Design review of the part built by this model. Coordinates are the model's own, in mm. A direction names the side the tool comes from. Coordinates: 2 decimals unless noted, no trailing zeros. Loops run counter-clockwise (first coordinate to the right, second up) from the corner with the lowest first, then second, coordinate; pieces in that order, holes last. Notation, with made-up numbers: (-36.75, 22) - (-4.75, 22) arc R18 ccw to (-4.75, 47) - close; hole circle Ø4 at (-36, 56.5). An arc over 180 degrees is marked (long way). Return JSON: item names as keys, results as strings. Group by question number.
from build123d import *

# Parameters (mm, degrees)
F0_R      = 2.4509487717
F1_DEPTH  = 4.7244
F2_R      = 19.05
F3_DEPTH  = 1.524
F5_DEPTH  = 2.54
F7_DEPTH  = 5.842
F8_DEPTH  = 52.9844
F9_DEPTH  = 10.795
F10_R     = 2.032
F12_R     = 3.81
F13_DEPTH = 75.8698
F16_R     = 3.81
F17_DEPTH = 63.5
F18_R     = 3.175
F19_DEPTH = 25.4
F21_DEPTH = 11.5824


with BuildPart() as f1:
    # F0 (on Top) → F1 (new body)
    with BuildSketch(Plane.XY):
        with BuildLine():
            Line((25.273, 28.575), (-25.273, 28.575))
            ThreePointArc((-25.273, 28.575), (-27.6078665915, 27.6078665915), (-28.575, 25.273))
            Line((-28.575, 25.273), (-28.575, -25.273))
            ThreePointArc((-28.575, -25.273), (-27.6078665915, -27.6078665915), (-25.273, -28.575))
            Line((-25.273, -28.575), (25.273, -28.575))
            ThreePointArc((25.273, -28.575), (27.6078665915, -27.6078665915), (28.575, -25.273))
            Line((28.575, -25.273), (28.575, 25.273))
            ThreePointArc((28.575, 25.273), (27.6078665915, 27.6078665915), (25.273, 28.575))
        make_face()
        with Locations((-23.495, -23.495)):
            Circle(F0_R, mode=Mode.SUBTRACT)
        with Locations((23.495, -23.495)):
            Circle(F0_R, mode=Mode.SUBTRACT)
        with Locations((-23.495, 23.495)):
            Circle(F0_R, mode=Mode.SUBTRACT)
        with Locations((23.495, 23.495)):
            Circle(F0_R, mode=Mode.SUBTRACT)
    extrude(amount=-F1_DEPTH)

    # F2 (on face) → F3 (join)
    with BuildSketch(Plane(origin=(0, 0, -4.7244), x_dir=(1, 0, 0), z_dir=(0, 0, -1))):
        Circle(F2_R)
    extrude(amount=F3_DEPTH)

    # F4 (on face) → F5 (cut)
    with BuildSketch(Plane(origin=(0, 0, -4.7244), x_dir=(1, 0, 0), z_dir=(0, 0, -1))):
        with BuildLine():
            Line((-28.575, 12.7), (-25.019, 12.7))
            ThreePointArc((-25.019, 12.7), (-22.098, 15.621), (-25.019, 18.542))
            Line((-25.019, 18.542), (-28.575, 18.542))
            Line((-28.575, 18.542), (-28.575, 12.7))
        make_face()
        with BuildLine():
            Line((28.575, -12.7), (25.019, -12.7))
            ThreePointArc((25.019, -12.7), (22.098, -15.621), (25.019, -18.542))
            Line((25.019, -18.542), (28.575, -18.542))
            Line((28.575, -18.542), (28.575, -12.7))
        make_face()
        with BuildLine():
            Line((12.7, 28.575), (12.7, 25.019))
            ThreePointArc((12.7, 25.019), (15.621, 22.098), (18.542, 25.019))
            Line((18.542, 25.019), (18.542, 28.575))
            Line((18.542, 28.575), (12.7, 28.575))
        make_face()
        with BuildLine():
            ThreePointArc((-12.7, -25.019), (-15.621, -22.098), (-18.542, -25.019))
            Line((-18.542, -25.019), (-18.542, -28.575))
            Line((-18.542, -28.575), (-12.7, -28.575))
            Line((-12.7, -28.575), (-12.7, -25.019))
        make_face()
    extrude(amount=-F5_DEPTH, mode=Mode.SUBTRACT)

    # F6 (on face) → F7 (join)
    with BuildSketch(Plane.XY):
        with BuildLine():
            Line((-21.717, 19.177), (-26.035, 19.177))
            ThreePointArc((-26.035, 19.177), (-27.8310512242, 18.4330512242), (-28.575, 16.637))
            Line((-28.575, 16.637), (-28.575, 0))
            Line((-28.575, 0), (-28.575, -16.637))
            ThreePointArc((-28.575, -16.637), (-27.8310512242, -18.4330512242), (-26.035, -19.177))
            Line((-26.035, -19.177), (-21.717, -19.177))
            ThreePointArc((-21.717, -19.177), (-19.9209487758, -19.9209487758), (-19.177, -21.717))
            Line((-19.177, -21.717), (-19.177, -26.035))
            ThreePointArc((-19.177, -26.035), (-18.4330512242, -27.8310512242), (-16.637, -28.575))
            Line((-16.637, -28.575), (16.637, -28.575))
            ThreePointArc((16.637, -28.575), (18.4330512242, -27.8310512242), (19.177, -26.035))
            Line((19.177, -26.035), (19.177, -21.717))
            ThreePointArc((19.177, -21.717), (19.9209487758, -19.9209487758), (21.717, -19.177))
            Line((21.717, -19.177), (26.035, -19.177))
            ThreePointArc((26.035, -19.177), (27.8310512242, -18.4330512242), (28.575, -16.637))
            Line((28.575, -16.637), (28.575, 0))
            Line((28.575, 0), (28.575, 16.637))
            ThreePointArc((28.575, 16.637), (27.8310512242, 18.4330512242), (26.035, 19.177))
            Line((26.035, 19.177), (21.717, 19.177))
            ThreePointArc((21.717, 19.177), (19.9209487758, 19.9209487758), (19.177, 21.717))
            Line((19.177, 21.717), (19.177, 26.035))
            ThreePointArc((19.177, 26.035), (18.4330512242, 27.8310512242), (16.637, 28.575))
            Line((16.637, 28.575), (-16.637, 28.575))
            ThreePointArc((-16.637, 28.575), (-18.4330512242, 27.8310512242), (-19.177, 26.035))
            Line((-19.177, 26.035), (-19.177, 21.717))
            ThreePointArc((-19.177, 21.717), (-19.9209487758, 19.9209487758), (-21.717, 19.177))
        make_face()
    extrude(amount=F7_DEPTH)

    # F8 (add): a face of the model
    f8_faces = [f1.faces().sort_by_distance(p)[0] for p in [
        (0, 0, 5.842),
    ]]
    extrude(f8_faces, amount=F8_DEPTH)

    # F9 (add): a face of the model
    f9_faces = [f1.faces().sort_by_distance(p)[0] for p in [
        (0, 0, 58.8264),
    ]]
    extrude(f9_faces, amount=F9_DEPTH)

    # F10
    f10_edges = [f1.edges().sort_by_distance(p)[0] for p in [
        (-28.575, 0, 69.6214),
    ]]
    fillet(f10_edges, radius=F10_R)

    # F12 (on face) → F13 (cut, through all)
    with BuildSketch(Plane(origin=(0, 0, -6.2484), x_dir=(1, 0, 0), z_dir=(0, 0, -1))):
        Circle(F12_R)
    extrude(amount=-F13_DEPTH, mode=Mode.SUBTRACT)

    # F16 (on offset) → F17 (join)
    with BuildSketch(Plane(origin=(0, 0, 1.3716), x_dir=(1, 0, 0), z_dir=(0, 0, -1))):
        Circle(F16_R)
    extrude(amount=-F17_DEPTH)

    # F18 (on offset) → F19 (join)
    with BuildSketch(Plane(origin=(0, 0, 1.3716), x_dir=(1, 0, 0), z_dir=(0, 0, -1))):
        Circle(F18_R)
    extrude(amount=F19_DEPTH)

    # F20 (on face) → F21 (cut)
    with BuildSketch(Plane(origin=(0, 0, -24.0284), x_dir=(1, 0, 0), z_dir=(0, 0, -1))):
        Polygon((-5.7085081935, 6.1885123141), (-5.7085081935, 2.667), (7.1385717019, 2.667), (7.1947467513, 2.667), (7.1947467513, 6.1885123141), align=None)
    extrude(amount=-F21_DEPTH, mode=Mode.SUBTRACT)


solid = f1.part
Item 1: For P1, Ø3, axis at x = -24, y = -16.5, coming from the -Z side; P2, Ø3.5, axis at x = 23.5, z = 26, coming from the +Y side; P3, Ø4, axis at x = -23.495, y = 23.495, coming from the +Z side; P4, Ø1.5, axis at x = -20, y = -4, coming from the -Z side, all flat-tipped, find the tip position at first contact; note any pin that passes through.
Item 2: Add section D-D (y = 11). State the section outline as (x, z) points (3 decimals).
Item 3: Add section C-C (z = 49). State the section outline as (x, y) points (3 decimals).
Item 4: Add section B-B (y = 0). State the section outline as (x, z) points (3 decimals), then the cut area to 3 significant figures.
Item 5: Add section A-A (x = 0). State the section outline as (y, z) points (3 decimals).
Item 6: Draft analysis for pull direction X (two halves, no side actions). For faces 5 (the face through (0, 0, 64.872)), 6 (the face through (-27, -12.7, -3)), 7 (the face through (27.582, -27.633, -2.329)), state which applies: pulls with the +X half, pulls with the -X half, needs draft (parallel to the pull), parting line crosses it, or undercut.
Item 7: To check wall thickness, follow line 1 (X direction, y = 0, z = -2.25) (3 decimals); line 2 (X direction, y = 0, z = 66) (3 decimals); line 3 (Z direction, x = 0, y = -11). State the ranges of each line that lie inside material, in increasing order. Write a range as from..to.
Item 8: For faces 1 (the face through (23.91, -18.6, 69.01)), 2 (the face through (-23.91, 18.6, 69.01)), 3 (the face through (-18.542, 27, -3)), 4 (the face through (18.6, 23.91, 69.01)), list the 3-axis set-ups (+Z, -Z, +X, -X, +Y, -Y) from which the entire face can be reached by the end or side of a thin tool; tool diameter is ignored.
Answers below:
{
 "1": {"P1": "stops at z = -2.18", "P2": "stops at y = 19.18", "P3": "passes through", "P4": "stops at z = -4.72"},
 "2": {"outline": "(-28.575, -4.724) - (-15.553, -4.724) - (-15.553, -6.248) - (15.553, -6.248) - (15.553, -4.724) - (28.575, -4.724) - (28.575, 67.589) arc R2.032 ccw to (26.543, 69.621) - (-26.543, 69.621) arc R2.032 ccw to (-28.575, 67.589) - close"},
 "3": {"outline": "(-28.575, -16.637) arc R2.54 ccw to (-26.035, -19.177) - (-21.717, -19.177) arc R2.54 cw to (-19.177, -21.717) - (-19.177, -26.035) arc R2.54 ccw to (-16.637, -28.575) - (16.637, -28.575) arc R2.54 ccw to (19.177, -26.035) - (19.177, -21.717) arc R2.54 cw to (21.717, -19.177) - (26.035, -19.177) arc R2.54 ccw to (28.575, -16.637) - (28.575, 16.637) arc R2.54 ccw to (26.035, 19.177) - (21.717, 19.177) arc R2.54 cw to (19.177, 21.717) - (19.177, 26.035) arc R2.54 ccw to (16.637, 28.575) - (-16.637, 28.575) arc R2.54 ccw to (-19.177, 26.035) - (-19.177, 21.717) arc R2.54 cw to (-21.717, 19.177) - (-26.035, 19.177) arc R2.54 ccw to (-28.575, 16.637) - close"},
 "4": {"outline": "(-28.575, -4.724) - (-19.05, -4.724) - (-19.05, -6.248) - (-3.81, -6.248) - (-3.81, 1.372) - (-3.175, 1.372) - (-3.175, -24.028) - (3.175, -24.028) - (3.175, 1.372) - (3.81, 1.372) - (3.81, -6.248) - (19.05, -6.248) - (19.05, -4.724) - (28.575, -4.724) - (28.575, 67.589) arc R2.032 ccw to (26.543, 69.621) - (3.81, 69.621) - (3.81, 64.872) - (-3.81, 64.872) - (-3.81, 69.621) - (-26.543, 69.621) arc R2.032 ccw to (-28.575, 67.589) - close", "area": "4,370 mm^2"},
 "5": {"outline": "(-28.575, -4.724) - (-19.05, -4.724) - (-19.05, -6.248) - (-3.81, -6.248) - (-3.81, 1.372) - (-3.175, 1.372) - (-3.175, -12.446) - (-2.667, -12.446) - (-2.667, -24.028) - (3.175, -24.028) - (3.175, 1.372) - (3.81, 1.372) - (3.81, -6.248) - (19.05, -6.248) - (19.05, -4.724) - (28.575, -4.724) - (28.575, 67.589) arc R2.032 ccw to (26.543, 69.621) - (3.81, 69.621) - (3.81, 64.872) - (-3.81, 64.872) - (-3.81, 69.621) - (-26.543, 69.621) arc R2.032 ccw to (-28.575, 67.589) - close"},
 "6": {"face 5": "undercut", "face 6": "needs draft", "face 7": "pulls with the +X half"},
 "7": {"line 1": "x = -28.575..-3.81, -3.175..3.175, 3.81..28.575", "line 2": "x = -28.575..-3.81, 3.81..28.575", "line 3": "z = -6.25..69.62"},
 "8": {"face 1": "+Z, +X, -Y", "face 2": "+Z, -X, +Y", "face 3": "-Z, +Y", "face 4": "+Z, +X, +Y"}
}
